```python
from build123d import *

# Parameters (mm, degrees)
F0_W     = 90
F0_H     = 60
F1_DEPTH = 50
F2_W     = 40
F2_H     = 20
F3_DEPTH = 50.001
F4_DEPTH = 50.001
F5_W     = 30
F5_H     = 15
F6_DEPTH = 60.001


with BuildPart() as f1:
    # F0 (on Front) → F1 (new body)
    with BuildSketch(Plane.XZ):
        Rectangle(F0_W, F0_H)
    extrude(amount=F1_DEPTH)

    # F2 (on face) → F3 (cut, through all)
    with BuildSketch(Plane.XZ.offset(50)):
        with Locations((25, 20)):
            Rectangle(F2_W, F2_H)
    extrude(amount=-F3_DEPTH, mode=Mode.SUBTRACT)

    # F2 (on face) → F4 (cut, through all)
    with BuildSketch(Plane.XZ.offset(50)):
        with Locations((25, -20)):
            Rectangle(F2_W, F2_H)
    extrude(amount=-F4_DEPTH, mode=Mode.SUBTRACT)

    # F5 (on face) → F6 (cut, through all)
    with BuildSketch(Plane.XY.offset(30)):
        with Locations((-30, -7.5)):
            Rectangle(F5_W, F5_H)
        with Locations((-30, -42.5)):
            Rectangle(F5_W, F5_H)
    extrude(amount=-F6_DEPTH, mode=Mode.SUBTRACT)


solid = f1.part
```
Work out the finished part from the listing and answer in its coordinate system (mm). A direction names the side the tool comes from. Give positions to 0.01 mm unless a question says otherwise; leave off trailing zeros. Loops run counter-clockwise (first coordinate to the right, second up) from the corner with the lowest first, then second, coordinate; pieces in that order, holes last. Notation, with made-up numbers: (3, -35) -> (38, -35) arc R7 cw to (38, -27) -> close; hole circle Ø5 at (-0.75, -12). An arc over 180 degrees is marked (long way). Write item = value, one per line. Start each with the question number.
(1) Find the intervals of material crossed by probe 1 along X at (y, z) = (-43.5, 11); probe 2 along Z at (x, y) = (32.5, -44.5); probe 3 along X at (y, z) = (-18.5, -22), in increasing order. Write a range as from..to.
(2) Find section D-D on x = 31. Give the vertices of the cut face in (y, z), and give its area (3 significant figures).
(3) Find section C-C on x = -32. Give the vertices of the cut face in (y, z).
(4) Given pin 1 Ø6 at (x, z) = (-24.5, -2) entering from -Y; pin 2 Ø15 at (x, z) = (-24, -14) entering from +Y; pin 3 Ø6 at (y, z) = (-34.5, -24) entering from +X, each flat-ended and moving along its own axis, determine where each tip first touches the part or whether it passes through.
(5) Which of the six approach directions +Z, -Z, +X, -X, +Y, -Y give full straight-line access (tool end or side, diameter ignored) to faces 1 (the flat face through (25, -25, 10)), 2 (the flat face through (-15, -8, 0)), 3 (the flat face through (-15, -43, 0))?
(6) Find section B-B on y = -44.5. Give the vertices of the cut face in (x, z), and give its area (3 significant figures).
(7) Find section A-A on z = -19. Give the vertices of the cut face in (x, y), and give its area (3 significant figures).
From the geometry:
q1.probe_1 = -15..5
q1.probe_2 = -10..10
q1.probe_3 = -45..5
q2.outline = (-50, -10) -> (0, -10) -> (0, 10) -> (-50, 10) -> close
q2.area = 1,000 mm^2
q3.outline = (-35, -30) -> (-15, -30) -> (-15, 30) -> (-35, 30) -> close
q4.pin_1 = -35
q4.pin_2 = -15
q4.pin_3 = 5
q5.face_1 = +Z, +X, +Y, -Y
q5.face_2 = +Z, -Z, -X, +Y
q5.face_3 = +Z, -Z, -X, -Y
q6.outline = (-15, -30) -> (5, -30) -> (5, -10) -> (45, -10) -> (45, 10) -> (5, 10) -> (5, 30) -> (-15, 30) -> close
q6.area = 2,000 mm^2
q7.outline = (-45, -35) -> (-15, -35) -> (-15, -50) -> (5, -50) -> (5, 0) -> (-15, 0) -> (-15, -15) -> (-45, -15) -> close
q7.area = 1,600 mm^2
